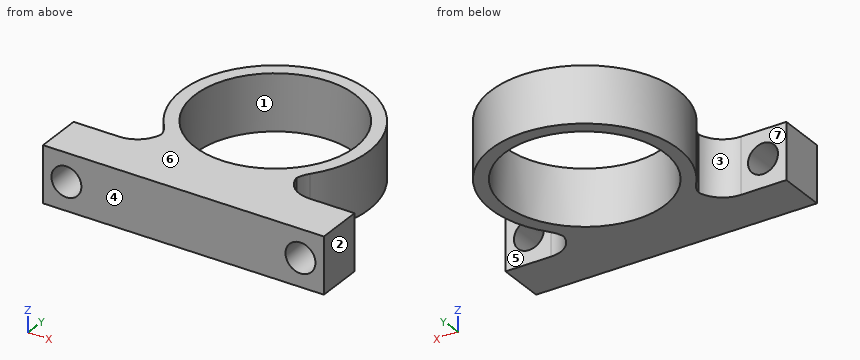
```python
from build123d import *

# Parameters (mm, degrees)
IZIM1_R                     = 10
IZIM1_R_2                   = 8.575
IZIM1_W                     = 30
IZIM1_H                     = 5
Y_KSEKLIK_EKSTR_ZYON1_DEPTH = 6
RADYUS1_R                   = 3
IZIM3_R                     = 1.6
KES_EKSTR_ZYON1_DEPTH       = 6
IZIM2_R                     = 1.6
KES_EKSTR_ZYON2_DEPTH       = 6


with BuildPart() as part:
    # Çizim1 → Yükseklik-Ekstrüzyon1 (new body)
    # profile 1 of 4: a face of its own
    with BuildSketch(Plane.XY):
        with Locations((0, 12.5)):
            Circle(IZIM1_R)
        with Locations((0, 12.5)):
            Circle(IZIM1_R_2, mode=Mode.SUBTRACT)
    # profile 2 of 4: a face of its own
    with BuildSketch(Plane.XY):
        with BuildLine():
            ThreePointArc((7.141428429, 5.5), (3.872983346, 3.280455543), (0, 2.5))
            Line((0, 2.5), (7.141428429, 2.5))
            Line((7.141428429, 2.5), (7.141428429, 5.5))
        make_face()
    # profile 3 of 4: a face of its own
    with BuildSketch(Plane.XY):
        with BuildLine():
            Line((-7.141428429, 5.5), (-7.141428429, 2.5))
            Line((-7.141428429, 2.5), (0, 2.5))
            ThreePointArc((0, 2.5), (-3.872983346, 3.280455543), (-7.141428429, 5.5))
        make_face()
    # profile 4 of 4: a face of its own
    with BuildSketch(Plane.XY):
        Rectangle(IZIM1_W, IZIM1_H)
    extrude(amount=Y_KSEKLIK_EKSTR_ZYON1_DEPTH)

    # Radyus1
    # the kernel refuses this fillet: 3 mm, written as the material it adds along each edge
    with BuildSketch(Plane(origin=(-7.141428429, 2.5, 0), x_dir=(-1, 0, 0), z_dir=(0, 0, 1))) as radyus1_piece_1:
        with BuildLine():
            CenterArc((RADYUS1_R, -RADYUS1_R), RADYUS1_R, 90, 90)
            Line((0, -RADYUS1_R), (0, 0))
            Line((0, 0), (RADYUS1_R, 0))
        make_face()
    extrude(amount=6)
    with BuildSketch(Plane(origin=(-7.141428429, 5.5, 0), x_dir=(0, -1, 0), z_dir=(0, 0, 1))) as radyus1_piece_2:
        with BuildLine():
            CenterArc((1.133352902, -3), RADYUS1_R, 90, 38.729363069)
            ThreePointArc((-0.743574691, -0.659670363), (-0.363585739, -0.33907996), (0, 0))
            Line((0, 0), (1.133352902, 0))
        make_face()
    extrude(amount=6)
    with BuildSketch(Plane(origin=(7.141428429, 5.5, 0), x_dir=(0, -1, 0), z_dir=(0, 0, 1))) as radyus1_piece_3:
        with BuildLine():
            CenterArc((1.133352902, 3), RADYUS1_R, 231.270636931, 38.729363069)
            ThreePointArc((-0.743574691, 0.659670363), (-0.363585739, 0.33907996), (0, 0))
            Line((0, 0), (1.133352902, 0))
        make_face()
    extrude(amount=6)
    with BuildSketch(Plane(origin=(7.141428429, 2.5, 0), x_dir=(1, 0, 0), z_dir=(0, 0, 1))) as radyus1_piece_4:
        with BuildLine():
            CenterArc((RADYUS1_R, RADYUS1_R), RADYUS1_R, 180, 90)
            Line((0, RADYUS1_R), (0, 0))
            Line((0, 0), (RADYUS1_R, 0))
        make_face()
    extrude(amount=6)

    # Çizim3 → Kes-Ekstrüzyon1 (cut)
    with BuildSketch(Plane(origin=(0, 2.5, 0), x_dir=(1, 0, 0), z_dir=(0, 1, 0))):
        with Locations(Location((12.5, -3, 0), (0, 0, 270))):
            Circle(IZIM3_R)
    extrude(amount=-KES_EKSTR_ZYON1_DEPTH, mode=Mode.SUBTRACT)

    # Çizim2 → Kes-Ekstrüzyon2 (cut)
    with BuildSketch(Plane(origin=(0, 2.5, 0), x_dir=(1, 0, 0), z_dir=(0, 1, 0))):
        with Locations(Location((-12.5, -3, 0), (0, 0, 270))):
            Circle(IZIM2_R)
    extrude(amount=-KES_EKSTR_ZYON2_DEPTH, mode=Mode.SUBTRACT)


solid = part.part
```
The model under review builds one solid part; all positions refer to its coordinate system, in mm. Face numbers are marked on the shaded views. A direction names the side the tool comes from. Give positions to 0.01 mm unless a question says otherwise; leave off trailing zeros. Write each loop counter-clockwise with the first axis right and the second up, starting at its lowest first coordinate (ties: lowest second). Pieces come first, ordered by that corner, then holes. Notation, with made-up numbers: (-33.75, 18.25) - (3.25, 18.25) arc R14 cw to (3.25, 34.25) - close; hole circle Ø3 at (41.5, -36.75). An arc over 180 degrees is marked (long way). Answer in a Markdown table with one row per item. Add a question column.
1. We need section A-A on x = -12.5. Write out the cut boundary in (y, z), then the cut area to 3 significant figures.
2. Insertion check: P1, Ø1.5, axis at y = 6, z = 3, coming from the +X side; P2, Ø3, axis at x = -9.5, z = 3, coming from the +Y side; P3, Ø2, axis at y = 4, z = 4.5, coming from the -X side; P4, Ø3, axis at x = -12.5, z = 3, coming from the +Y side. Each pin has a flat end and moves straight along its axis. Give the tip position at first contact, or say it passes through.
3. We need section C-C on z = 3. Write out the cut boundary in (x, y) (3 decimals), then the cut area to 3 significant figures.
4. Draft analysis for pull direction X (two halves, no side actions). For the marked faces 1, 2, 3 and 4, state which applies: +X half, -X half, draft (parallel to the pull), parting line (faces both ways), or undercut.
5. We need section D-D on z = 0.4. Write out the cut boundary in (x, y) (3 decimals).
6. Wall thickness on line 1 along X through (y, z) = (1.45, 3); line 2 along Y through (x, z) = (7.75, 4.95); line 3 along Y through (x, z) = (-7.5, 5.25): over which ranges is each line inside the solid? List them lowest first. Write a range as [from, to].
7. Tool access review of the marked faces 5, 6 and 7: name each direction out of +Z, -Z, +X, -X, +Y, -Y from which nothing blocks a thin tool from reaching the whole face with its end or side.
8. We need section B-B on y = 12.5. Write out the cut boundary in (x, z) (3 decimals), then the cut area to 3 significant figures.
Ans:
| question | item | result |
|---|---|---|
| 1 | outline | (-2.5, 0) - (2.5, 0) - (2.5, 1.4) - (-2.5, 1.4) - close; (-2.5, 4.6) - (2.5, 4.6) - (2.5, 6) - (-2.5, 6) - close |
| 1 | area | 14.0 mm^2 |
| 2 | P1 | stops at x = 8.18 |
| 2 | P2 | stops at y = 18.5 |
| 2 | P3 | stops at x = -8.48 |
| 2 | P4 | passes through |
| 3 | outline | (-15, -2.5) - (-14.1, -2.5) - (-14.1, 2.5) - (-15, 2.5) - close; (-10.9, -2.5) - (10.9, -2.5) - (10.9, 2.5) - (10.141, 2.5) arc R3 cw to (7.195, 4.933) arc R3 cw to (7.801, 6.244) arc R10 ccw (long way) to (-7.801, 6.244) arc R3 cw to (-7.195, 4.933) arc R3 cw to (-10.141, 2.5) - (-10.9, 2.5) - close; (14.1, -2.5) - (15, -2.5) - (15, 2.5) - (14.1, 2.5) - close; hole circle Ø17.15 at (0, 12.5) |
| 3 | area | 219 mm^2 |
| 4 | face 1 | undercut |
| 4 | face 2 | +X half |
| 4 | face 3 | -X half |
| 4 | face 4 | draft |
| 5 | outline | (-15, -2.5) - (15, -2.5) - (15, 2.5) - (10.141, 2.5) arc R3 cw to (7.195, 4.933) arc R3 cw to (7.801, 6.244) arc R10 ccw (long way) to (-7.801, 6.244) arc R3 cw to (-7.195, 4.933) arc R3 cw to (-10.141, 2.5) - (-15, 2.5) - close; hole circle Ø17.15 at (0, 12.5) |
| 6 | line 1 | x = [-15, -14.1], [-10.9, 10.9], [14.1, 15] |
| 6 | line 2 | y = [-2.5, 3.69], [6.18, 8.83], [16.17, 18.82] |
| 6 | line 3 | y = [-2.5, 4.08], [5.79, 8.34], [16.66, 19.11] |
| 7 | face 5 | +Z, -Z, +X, +Y |
| 7 | face 6 | +Z, +X, -X, +Y, -Y |
| 7 | face 7 | +Z, -Z, -X, +Y |
| 8 | outline | (-10, 0) - (-8.575, 0) - (-8.575, 6) - (-10, 6) - close; (8.575, 0) - (10, 0) - (10, 6) - (8.575, 6) - close |
| 8 | area | 17.1 mm^2 |
